Read the model definition and answer for the solid it produces. Units are mm, in the model's axes. A direction names the side the tool comes from. Coordinates: 2 decimals unless noted, no trailing zeros. Loops run counter-clockwise (first coordinate to the right, second up) from the corner with the lowest first, then second, coordinate; pieces in that order, holes last.
from build123d import *

# Parameters (mm, degrees)
ESQUISSE1_W          = 14
ESQUISSE1_H          = 16.9
BASE_EXTRUSION_DEPTH = 9
ESQUISSE2_R          = 1.35
BOSS_EXTRU_1_DEPTH   = 7.9
ESQUISSE3_R          = 1.35
BOSS_EXTRU_2_DEPTH   = 6
EXTRUSION1_DEPTH     = 0.9
EXTRUSION2_DEPTH     = 0.9


with BuildPart() as part:
    # Esquisse1 → Base-Extrusion (new body)
    with BuildSketch(Plane.XY):
        with Locations((7, 8.45)):
            Rectangle(ESQUISSE1_W, ESQUISSE1_H)
    extrude(amount=BASE_EXTRUSION_DEPTH)

    # Esquisse2 → Boss.-Extru.1 (add)
    with BuildSketch(Plane.XZ):
        with Locations(Location((7, 1.8, 0), (0, 0, 90))):
            Circle(ESQUISSE2_R)
    extrude(amount=BOSS_EXTRU_1_DEPTH)

    # Esquisse3 → Boss.-Extru.2 (add)
    with BuildSketch(Plane.XZ):
        with Locations((3.7, 9.921362126)):
            Circle(ESQUISSE3_R)
    extrude(amount=-BOSS_EXTRU_2_DEPTH)

    # Esquisse4 → Extrusion1 (add)
    with BuildSketch(Plane.ZY):
        Polygon((3.607457233, 13.98057371), (-1.5, 13.98057371), (-1.5, 13.53057371), (-4, 13.53057371), (-4, 12.93057371), (-1.5, 12.93057371), (-1.5, 12.48057371), (3.607457233, 12.48057371), align=None)
        Polygon((3.607457233, 10.68057371), (-1.5, 10.68057371), (-1.5, 10.23057371), (-4, 10.23057371), (-4, 9.63057371), (-1.5, 9.63057371), (-1.5, 9.18057371), (3.607457233, 9.18057371), align=None)
        Polygon((3.607457233, 7.38057371), (-1.5, 7.38057371), (-1.5, 6.93057371), (-4, 6.93057371), (-4, 6.33057371), (-1.5, 6.33057371), (-1.5, 5.88057371), (3.607457233, 5.88057371), align=None)
        Polygon((3.607457233, 4.08057371), (-1.5, 4.08057371), (-1.5, 3.63057371), (-4, 3.63057371), (-4, 3.03057371), (-1.5, 3.03057371), (-1.5, 2.58057371), (3.607457233, 2.58057371), align=None)
    extrude(amount=EXTRUSION1_DEPTH)

    # Esquisse5 → Extrusion2 (add)
    with BuildSketch(Plane(origin=(14, 0, 0), x_dir=(0, 0, -1), z_dir=(1, 0, 0))):
        Polygon((1.5, 13.98057371), (-3.607457233, 13.98057371), (-3.607457233, 12.48057371), (1.5, 12.48057371), (1.5, 12.93057371), (4, 12.93057371), (4, 13.53057371), (1.5, 13.53057371), align=None)
        Polygon((1.5, 7.38057371), (-3.607457233, 7.38057371), (-3.607457233, 5.88057371), (1.5, 5.88057371), (1.5, 6.33057371), (4, 6.33057371), (4, 6.93057371), (1.5, 6.93057371), align=None)
        Polygon((-3.607457233, 10.68057371), (-3.607457233, 9.18057371), (1.5, 9.18057371), (1.5, 9.63057371), (4, 9.63057371), (4, 10.23057371), (1.5, 10.23057371), (1.5, 10.68057371), align=None)
        Polygon((-3.607457233, 4.08057371), (-3.607457233, 2.58057371), (1.5, 2.58057371), (1.5, 3.03057371), (4, 3.03057371), (4, 3.63057371), (1.5, 3.63057371), (1.5, 4.08057371), align=None)
    extrude(amount=EXTRUSION2_DEPTH)


solid = part.part
Item 1: Given pin 1 (2 mm diameter, centred on x = 5, z = 6, fed in from -Y); pin 2 (0.5 mm diameter, centred on x = 14.5, z = -2.5, fed in from -Y); pin 3 (4 mm diameter, centred on x = 10.5, y = -4.5, fed in from +Z); pin 4 (2 mm diameter, centred on y = 12.5, z = 5.5, fed in from -X), each flat-ended and moving along its own axis, determine where each tip first touches the part or whether it passes through.
Numbers:
pin 1: stops at y = 0
pin 2: stops at y = 3.03
pin 3: passes through
pin 4: stops at x = 0
Item 2: A cutting plane is placed at D-D on x = 3.7. Determine the outline of the cut face in (y, z), then the cut area to 3 significant figures.
Numbers:
outline: (0, 0) - (16.9, 0) - (16.9, 9) - (6, 9) - (6, 11.27) - (0, 11.27) - close
area: 166 mm2
Item 3: Find the intervals of material crossed by line 1 along X through (y, z) = (0.25, 5.5); line 2 along Y through (x, z) = (4.5, 9.25); line 3 along Y through (x, z) = (8, 2.75), in increasing order.
Numbers:
line 1: x = 0 to 14
line 2: y = 0 to 6
line 3: y = 0 to 16.9
Item 4: A cutting plane is placed at B-B on x = 7. Determine the outline of the cut face in (y, z), then the cut area to 3 significant figures.
Numbers:
outline: (-7.9, 0.45) - (0, 0.45) - (0, 0) - (16.9, 0) - (16.9, 9) - (0, 9) - (0, 3.15) - (-7.9, 3.15) - close
area: 173 mm2
Item 5: A cutting plane is placed at A-A on z = -2.75. Give the number of separate pieces and of enclosed holes in the cut face, then the cut area to 3 significant figures.
Numbers:
separate pieces: 8
enclosed holes: 0
area: 4.32 mm2
Item 6: A cutting plane is placed at C-C on y = -5.5. Determine the outline of the cut face in (x, z), then the cut area to 3 significant figures.
Numbers:
outline: circle Ø2.7 at (7, 1.8)
area: 5.73 mm2
Item 7: Determine the mould class of faces 1 (the face through (-0.4, 13.531, -2.7)), 2 (the face through (14.9, 10, 1)), 3 (the face through (14.4, 4.081, 1)) for opening direction Y: released by +Y, released by -Y, zero draft, split by the parting line, or undercut.
Numbers:
face 1: released by +Y
face 2: zero draft
face 3: undercut
Item 8: Which of the six approach directions +Z, -Z, +X, -X, +Y, -Y give full straight-line access (tool end or side, diameter ignored) to faces 4 (the face through (-0.4, 9.181, 1)), 5 (the face through (14.4, 3.631, -2.8)), 6 (the face through (14.4, 13.531, -2.8))?
Numbers:
face 4: +Z, -Z, -X
face 5: -Z, +X, -X
face 6: -Z, +X, -X, +Y
